Check sheet for the modelled part. Datum: model origin and axes. Units: mm. Give positions to 0.01 mm unless a question says otherwise; leave off trailing zeros. Write each loop counter-clockwise with the first axis right and the second up, starting at its lowest first coordinate (ties: lowest second). Pieces come first, ordered by that corner, then holes.
from build123d import *

# Parameters (mm, degrees)
SKETCH_1_W          = 80
SKETCH_1_H          = 10
EXTRUDE_1_DEPTH     = 2
SKETCH_2_R          = 1
CUT_EXTRUDE_1_DEPTH = 2
SKETCH_5_R          = 5.1
CUT_EXTRUDE_2_DEPTH = 1.2


with BuildPart() as part:
    # 草图1 → 凸台-拉伸1 (new body)
    with BuildSketch(Plane(origin=(0, 0, 0), x_dir=(0, 0, -1), z_dir=(1, 0, 0))):
        with Locations((-40, 5)):
            Rectangle(SKETCH_1_W, SKETCH_1_H)
    extrude(amount=EXTRUDE_1_DEPTH)

    # 草图2 → 切除-拉伸1 (cut)
    with BuildSketch(Plane(origin=(2, 0, 0), x_dir=(0, 0, -1), z_dir=(1, 0, 0))):
        with Locations((-76, 5)):
            Circle(SKETCH_2_R)
        with Locations((-4, 5)):
            Circle(SKETCH_2_R)
    extrude(amount=-CUT_EXTRUDE_1_DEPTH, mode=Mode.SUBTRACT)

    # 草图5 → 切除-拉伸2 (cut)
    with BuildSketch(Plane(origin=(2, 0, 0), x_dir=(0, 0, -1), z_dir=(1, 0, 0))):
        with Locations((-68, 5)):
            Circle(SKETCH_5_R)
        with Locations((-12, 5)):
            Circle(SKETCH_5_R)
    extrude(amount=-CUT_EXTRUDE_2_DEPTH, mode=Mode.SUBTRACT)


solid = part.part
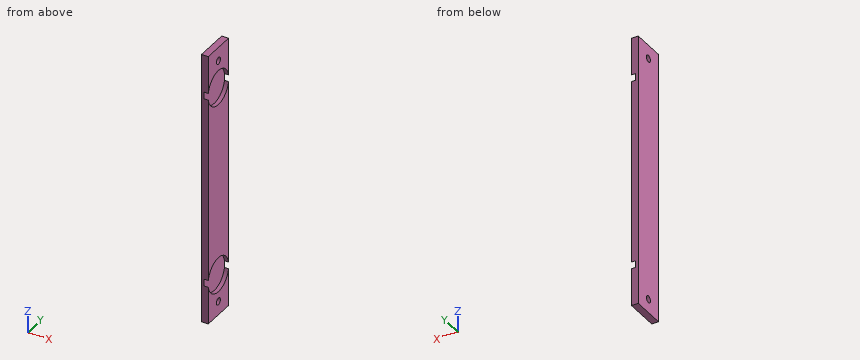
1) Sectioned sample at C-C on y = 8.25. Record the boundary of the cut face in (x, z).
2) Gauge pin test, flat end, axial feed: pin 1 (1.8 mm diameter, centred on y = 5, z = 76, fed in from -X). Record the tip position at first contact, or that the pin passes through.
3) Sectioned sample at A-A on x = 1.65. Record the boundary of the cut face in (y, z), then the cut area to 3 significant figures.
4) Sectioned sample at B-B on z = 4. Record the boundary of the cut face in (x, y), then the cut area to 3 significant figures.
5) Scan lines: L1, parallel to Y at x = 1.55, z = 76; L2, parallel to Z at x = 1.5, y = 6.25; L3, parallel to Z at x = 0.5, y = 4.25. Record each from-to range of solid material in increasing order.
6) Sectioned sample at D-D on z = 72. Record the boundary of the cut face in (x, y).
Answers below:
1. outline: (0, 0) - (2, 0) - (2, 8.07) - (0.8, 8.07) - (0.8, 15.93) - (2, 15.93) - (2, 64.07) - (0.8, 64.07) - (0.8, 71.93) - (2, 71.93) - (2, 80) - (0, 80) - close
2. pin 1: passes through
3. outline: (0, 0) - (10, 0) - (10, 11) arc R5.1 cw to (0, 11) - close; (0, 13) arc R5.1 cw to (10, 13) - (10, 67) arc R5.1 cw to (0, 67) - close; (0, 69) arc R5.1 cw to (10, 69) - (10, 80) - (0, 80) - close; hole circle Ø2 at (5, 4); hole circle Ø2 at (5, 76)
3. area: 631 mm2
4. outline: (0, 0) - (2, 0) - (2, 4) - (0, 4) - close; (0, 6) - (2, 6) - (2, 10) - (0, 10) - close
4. area: 16.0 mm2
5. L1: y = 0 to 4, 6 to 10
5. L2: z = 0 to 7.06, 16.94 to 63.06, 72.94 to 80
5. L3: z = 0 to 3.34, 4.66 to 75.34, 76.66 to 80
6. outline: (0, 0) - (2, 0) - (2, 1.84) - (0.8, 1.84) - (0.8, 8.16) - (2, 8.16) - (2, 10) - (0, 10) - close
